```python
from build123d import *

# Parameters (mm, degrees)
F0_W      = 35
F0_H      = 28.4
F1_DEPTH  = 12
F3_DEPTH  = 5
F5_DEPTH  = 5
F7_DEPTH  = 36.3
F8_W      = 24
F8_H      = 20
F9_DEPTH  = 8.5
F10_R     = 3.25
F11_DEPTH = 25
F13_DEPTH = 28.4


with BuildPart() as f1:
    # F0 (on Top) → F1 (new body)
    with BuildSketch(Plane.XY):
        Rectangle(F0_W, F0_H)
    extrude(amount=F1_DEPTH)

    # F2 (on face) → F3 (cut)
    with BuildSketch(Plane.XZ.offset(14.2)):
        Polygon((15, 8), (17.5, 0), (17.5, 8), align=None)
    extrude(amount=-F3_DEPTH, mode=Mode.SUBTRACT)

    # F4 (on face) → F5 (cut)
    with BuildSketch(Plane(origin=(0, 14.2, 0), x_dir=(-1, 0, 0), z_dir=(0, 1, 0))):
        Polygon((-15, 8), (-17.5, 8), (-17.5, 0), align=None)
    extrude(amount=-F5_DEPTH, mode=Mode.SUBTRACT)

    # F6 (on face) → F7 (cut)
    with BuildSketch(Plane(origin=(0, 14.2, 0), x_dir=(-1, 0, 0), z_dir=(0, 1, 0))):
        Polygon((12.5, 8), (17.5, 0), (17.5, 8), align=None)
    extrude(amount=-F7_DEPTH, mode=Mode.SUBTRACT)

    # F8 (on face) → F9 (cut)
    with BuildSketch(Plane(origin=(0, 0, 0), x_dir=(1, 0, 0), z_dir=(0, 0, -1))):
        Rectangle(F8_W, F8_H)
    extrude(amount=-F9_DEPTH, mode=Mode.SUBTRACT)

    # F10 (on face) → F11 (cut)
    with BuildSketch(Plane(origin=(0, 0, 8.5), x_dir=(1, 0, 0), z_dir=(0, 0, -1))):
        Circle(F10_R)
    extrude(amount=-F11_DEPTH, mode=Mode.SUBTRACT)

    # F12 (on face) → F13 (cut, through all)
    with BuildSketch(Plane(origin=(0, 14.2, 0), x_dir=(-1, 0, 0), z_dir=(0, 1, 0))):
        Polygon((17.25, 0), (17.5, 0), (17.25, 0.4), align=None)
    extrude(amount=-F13_DEPTH, mode=Mode.SUBTRACT)


solid = f1.part
```
For this review, take the finished solid that the model builds, in its own axes (mm). A direction names the side the tool comes from. Coordinates: 2 decimals unless noted, no trailing zeros. Write each loop counter-clockwise with the first axis right and the second up, starting at its lowest first coordinate (ties: lowest second). Pieces come first, ordered by that corner, then holes. Notation, with made-up numbers: (-29.5, 46.5) - (-19.5, 46.5) arc R20 cw to (-19.5, 74.5) - close; hole circle Ø11 at (80.5, 71.25). An arc over 180 degrees is marked (long way). Answer in a Markdown table with one row per item. Add a question column.
Q1. For probe 1 along X at (y, z) = (0, 10.65); probe 2 along Y at (x, z) = (0, 11.2); probe 3 along Y at (x, z) = (-10, 6.5), list the stretches that pass through material, from the lowest coordinate up.
Q2. We need section D-D, the plane x = 8. State the section outline as (y, z) points.
Q3. Draft analysis for pull direction X (two halves, no side actions). For faces 1 (the flat face through (-15, 0, 4)), 2 (the flat face through (16.23, -11.74, 4.06)), 3 (the cylindrical face through (-2.579, 1.978, 10.226)), state which applies: +X half, -X half, draft (parallel to the pull), parting line (faces both ways), or undercut.
Q4. We need section C-C, the plane z = 11.25. State the section outline as (x, y) points, and give its area (3 significant figures).
Q5. For P1, Ø10.5, axis at x = 0, y = 0, coming from the +Z side; P2, Ø10, axis at x = 2, y = -4.5, coming from the -Z side, all flat-tipped, find the tip position at first contact; note any pin that passes through.
Q6. We need section A-A, the plane x = -14. State the section outline as (y, z) points.
Q7. Tool access review of faces 4 (the flat face through (0, 10, 4)), 5 (the flat face through (0, 14.2, 6)), 6 (the flat face through (17, 9.2, 5)), 7 (the flat face through (16, -12, 8)), 8 (the flat face through (17.5, 0, 7)): name each direction out of +Z, -Z, +X, -X, +Y, -Y from which nothing blocks a thin tool from reaching the whole face with its end or side.
Q8. We need section B-B, the plane y = 0. State the section outline as (x, z) points.
Answer list:
| question | item | result |
|---|---|---|
| 1 | probe 1 | x = -17.5 to -3.25, 3.25 to 17.5 |
| 1 | probe 2 | y = -14.2 to -3.25, 3.25 to 14.2 |
| 1 | probe 3 | y = -14.2 to -10, 10 to 14.2 |
| 2 | outline | (-14.2, 0) - (-10, 0) - (-10, 8.5) - (10, 8.5) - (10, 0) - (14.2, 0) - (14.2, 12) - (-14.2, 12) - close |
| 3 | face 1 | -X half |
| 3 | face 2 | +X half |
| 3 | face 3 | undercut |
| 4 | outline | (-17.5, -14.2) - (17.5, -14.2) - (17.5, 14.2) - (-17.5, 14.2) - close; hole circle Ø6.5 at (0, 0) |
| 4 | area | 961 mm2 |
| 5 | P1 | stops at z = 12 |
| 5 | P2 | stops at z = 8.5 |
| 6 | outline | (-14.2, 0) - (14.2, 0) - (14.2, 5.6) - (-14.2, 5.6) - close; (-14.2, 8) - (14.2, 8) - (14.2, 12) - (-14.2, 12) - close |
| 7 | face 4 | -Z |
| 7 | face 5 | +Z, -Z, +X, -X, +Y |
| 7 | face 6 | +X, +Y |
| 7 | face 7 | +X, -Y |
| 7 | face 8 | +Z, -Z, +X, +Y, -Y |
| 8 | outline | (-17.5, 8) - (-12.5, 8) - (-17.25, 0.4) - (-17.25, 0) - (-12, 0) - (-12, 8.5) - (-3.25, 8.5) - (-3.25, 12) - (-17.5, 12) - close; (3.25, 8.5) - (12, 8.5) - (12, 0) - (17.5, 0) - (17.5, 12) - (3.25, 12) - close |
